For this review, use the dimensioned drawing (mm, ordinates from the lowest corner) and the shaded views. A direction names the side the tool comes from. Coordinates: 2 decimals unless noted, no trailing zeros. Loops run counter-clockwise (first coordinate to the right, second up) from the corner with the lowest first, then second, coordinate; pieces in that order, holes last. Notation, with made-up numbers: (-29, -28.75) - (29, -28.75) arc R18 cw to (29, -8.75) - close; hole circle Ø8 at (62, 59). An arc over 180 degrees is marked (long way). Use a Markdown table: item, result. Add a question column.
1) For the marked faces 1 and 2, list the 3-axis set-ups (+Z, -Z, +X, -X, +Y, -Y) from which the entire face can be reached by the end or side of a thin tool; tool diameter is ignored.
2) Clearance check with flat-ended pins moving along their axes: pin 1 (1.5 mm diameter, centred on y = 5.5, z = 16, fed in from -X); pin 2 (1.5 mm diameter, centred on y = 3, z = 22, fed in from -X); pin 3 (2 mm diameter, centred on x = 3, z = 20, fed in from -Y); pin 4 (3 mm diameter, centred on x = 4, y = 4, fed in from -Z). State where each tip first meets the part, or that it passes through.
3) Add section A-A, the plane z = 13. Give the boundary of the cut face in (x, y).
4) To check wall thickness, follow L1, parallel to Z at x = 1.25, y = 2; L2, parallel to X at y = 4.5, z = 12.5; L3, parallel to X at y = 3.5, z = 21.25. State the ranges of each line that lie inside material, in increasing order. Write a range as [from, to].
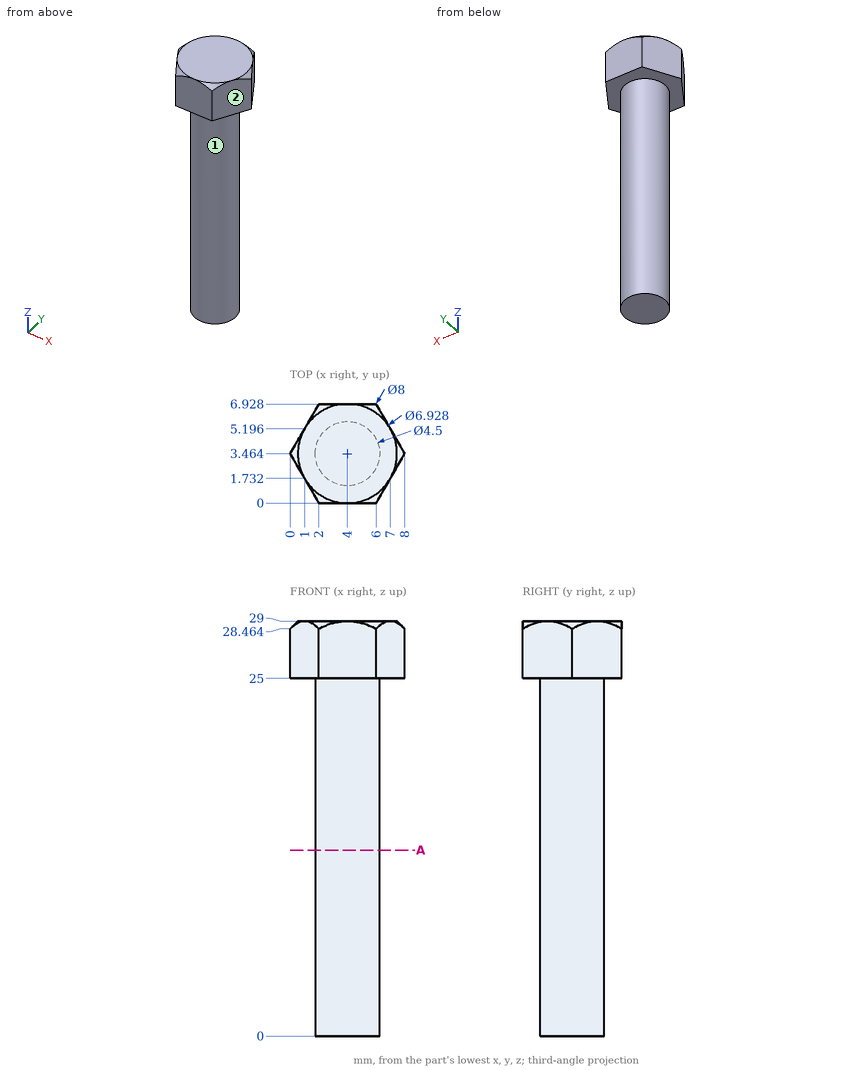
From the geometry:
| question | item | result |
|---|---|---|
| 1 | face 1 | -Z |
| 1 | face 2 | +Z, -Z, +X, -Y |
| 2 | pin 1 | stops at x = 2.15 |
| 2 | pin 2 | stops at x = 1.75 |
| 2 | pin 3 | stops at y = 1.21 |
| 2 | pin 4 | stops at z = 0 |
| 3 | outline | circle Ø4.5 at (4, 3.46) |
| 4 | L1 | z = [25, 29] |
| 4 | L2 | x = [2, 6] |
| 4 | L3 | x = [1.75, 6.25] |
